from build123d import *
from build123d.topology import SkipClean

# Parameters (mm, degrees)
BOSS_EXTRUDE1_DEPTH                = 7.5
CUT_EXTRUDE1_REACH                 = 158.924
SKETCH2_W                          = 18
SKETCH2_H                          = 40
M5_CLEARANCE_HOLE1_D               = 5.8
CUT_EXTRUDE2_REACH                 = 158.924
F_7_0_7_DIAMETER_HOLE1_D           = 7
F_7_0_7_DIAMETER_HOLE1_DEPTH       = 20
MOVE_FACE1_BY                      = 0.6
SKETCH15_W                         = 15
SKETCH15_H                         = 15
BOSS_EXTRUDE3_DEPTH                = 10
M5_CLEARANCE_HOLE2_D               = 5.8
SKETCH19_W                         = 125
SKETCH19_H                         = 15
SKETCH19_R                         = 3.5
SKETCH19_R_2                       = 5
BOSS_EXTRUDE4_DEPTH                = 6
SKETCH23_R                         = 5
SKETCH23_R_2                       = 2.9
BOSS_EXTRUDE5_DEPTH                = 1
F_4_5_START                        = -7.5
F_4_5_4_5_DIAMETER_HOLE1_OUTLINE_R = 2.25
F_4_5_4_5_DIAMETER_HOLE1_DEPTH     = 15


# Read off the part's stored shape, not the designer's step: Ø4.5 (4.5) Diameter Hole1
with BuildPart() as part:
    # Sketch1 → Boss-Extrude1 (new, symmetric)
    with BuildSketch(Plane.XY):
        Polygon((0, 0), (120, 0), (0, -100), align=None)
    extrude(amount=BOSS_EXTRUDE1_DEPTH, both=True)

    # Sketch2 → Cut-Extrude1 (cut, up to next)
    with BuildSketch(Plane.XY.offset(7.5), mode=Mode.PRIVATE) as cut_extrude1_sk1:
        with Locations((9, -40)):
            Rectangle(SKETCH2_W, SKETCH2_H)
    cut_extrude1_tool1 = extrude(cut_extrude1_sk1.sketch, amount=-CUT_EXTRUDE1_REACH, mode=Mode.PRIVATE) & part.part
    add(cut_extrude1_tool1.solids().sort_by_distance((9, -40, 7.5))[0], mode=Mode.SUBTRACT)

    # M5 Clearance Hole1 (through all)
    with Locations(Plane(origin=(0, 0, 0), x_dir=(1, 0, 0), z_dir=(0, 1, 0))):
        with Locations((4.5, 0)):
            Hole(M5_CLEARANCE_HOLE1_D / 2)

    # Sketch8 → Cut-Extrude2 (cut, up to next)
    with BuildSketch(Plane.XY.offset(7.5), mode=Mode.PRIVATE) as cut_extrude2_sk1:
        Polygon((0, -70), (36, -70), (0, -100), align=None)
    cut_extrude2_tool1 = extrude(cut_extrude2_sk1.sketch, amount=-CUT_EXTRUDE2_REACH, mode=Mode.PRIVATE) & part.part
    add(cut_extrude2_tool1.solids().sort_by_distance((12, -80, 7.5))[0], mode=Mode.SUBTRACT)

    # Ø7.0 (7) Diameter Hole1
    with Locations(Plane(origin=(0, 0, 0), x_dir=(1, 0, 0), z_dir=(0, 1, 0))):
        with Locations((115, 0)):
            Hole(F_7_0_7_DIAMETER_HOLE1_D / 2, depth=F_7_0_7_DIAMETER_HOLE1_DEPTH)

    # Move Face1: a curved face moved inward by 0.6
    add(Solid.thicken(part.faces().sort_by_distance((7.4, -65, 0))[0], -MOVE_FACE1_BY), mode=Mode.SUBTRACT)

    # Sketch15 → Boss-Extrude3 (add)
    with BuildSketch(Plane.ZY):
        with Locations((0, -77.5)):
            Rectangle(SKETCH15_W, SKETCH15_H)
    extrude(amount=-BOSS_EXTRUDE3_DEPTH)

    # M5 Clearance Hole2 (through all)
    with Locations(Plane(origin=(10, 0, 0), x_dir=(0, 0, -1), z_dir=(1, 0, 0))):
        with Locations((0, -77.5)):
            Hole(M5_CLEARANCE_HOLE2_D / 2)

    # Sketch19 → Boss-Extrude4 (add)
    with SkipClean():  # the faces are left unmerged after this step: merging them gives an invalid solid
        with BuildSketch(Plane(origin=(0, 0, 0), x_dir=(1, 0, 0), z_dir=(0, 1, 0))):
            with Locations((57.5, 0)):
                Rectangle(SKETCH19_W, SKETCH19_H)
            with Locations(Location((115, 0, 0), (0, 0, 270))):
                Circle(SKETCH19_R, mode=Mode.SUBTRACT)
            with Locations(Location((4.5, 0, 0), (0, 0, 154.158067237))):
                Circle(SKETCH19_R_2, mode=Mode.SUBTRACT)
        extrude(amount=BOSS_EXTRUDE4_DEPTH)

    # Sketch23 → Boss-Extrude5 (add)
    with BuildSketch(Plane(origin=(0, 0, 0), x_dir=(1, 0, 0), z_dir=(0, 1, 0))):
        with Locations(Location((4.5, 0, 0), (0, 0, 270))):
            Circle(SKETCH23_R)
        with Locations(Location((4.5, 0, 0), (0, 0, 270))):
            Circle(SKETCH23_R_2, mode=Mode.SUBTRACT)
    extrude(amount=BOSS_EXTRUDE5_DEPTH)

    # Ø4.5 (4.5) Diameter Hole1 outline → Ø4.5 (4.5) Diameter Hole1 (cut)
    with BuildSketch(Plane.XY.offset(F_4_5_START)):
        with Locations((91, -4)):
            Circle(F_4_5_4_5_DIAMETER_HOLE1_OUTLINE_R)
        with Locations((28, -57)):
            Circle(F_4_5_4_5_DIAMETER_HOLE1_OUTLINE_R)
        with Locations((28, -4)):
            Circle(F_4_5_4_5_DIAMETER_HOLE1_OUTLINE_R)
    extrude(amount=F_4_5_4_5_DIAMETER_HOLE1_DEPTH, mode=Mode.SUBTRACT)


solid = part.part
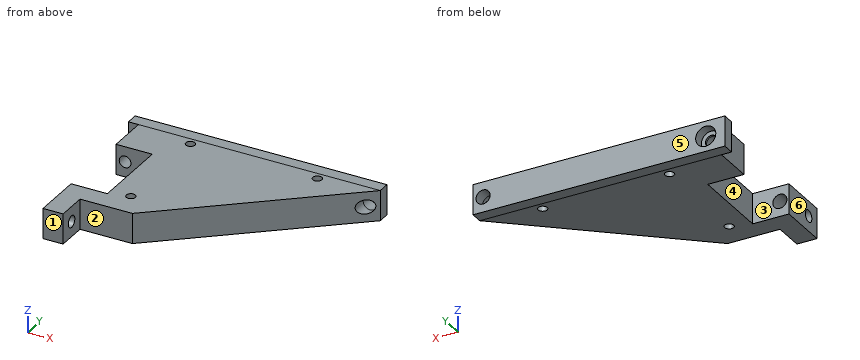
Can you work these out from the model? Positions are in its coordinate system, mm. Face numbers are marked on the shaded views. A direction names the side the tool comes from. Coordinates: 2 decimals unless noted, no trailing zeros. Loops run counter-clockwise (first coordinate to the right, second up) from the corner with the lowest first, then second, coordinate; pieces in that order, holes last. Notation, with made-up numbers: (53.25, -39.75) - (65.25, -39.75) arc R17 cw to (65.25, -17.75) - close; hole circle Ø5 at (-39, -29). An arc over 180 degrees is marked (long way). Put each result on its own line as item: value. Start each with the question number.
Item 1: Suppose I cut it at C-C (x = 3). Please give me the cut outline in (y, z), and give its area (3 significant figures).
Item 2: Suppose I cut it at B-B (x = 28). Please give me the cut outline in (y, z).
Item 3: If I drill on line 1 along X through (y, z) = (0.8, 0); line 2 along Y through (x, z) = (7, -5.25); line 3 along Z through (x, y) = (4.5, 4.75), over which ranges is the centre line in solid material (lowest first)?
Item 4: If we mould it in two halves opening along Y, with no side actions, what happens to the marked faces 3, 4, 5 and 6? For each: +Y half, -Y half, draft (parallel to the pull), parting line (faces both ways), or undercut.
Item 5: Which directions (+Z, -Z, +X, -X, +Y, -Y) give clear straight access to the entire face, cutting with the end or side of a thin tool? Please do the marked faces 1 and 2.
Item 6: Suppose I cut it at A-A (y = -57). Please give me the cut outline in (x, z), and give its area (4 significant figures).
Item 7: For pin 1 (4.5 mm diameter, centred on y = -76, z = 1, fed in from -X); pin 2 (3 mm diameter, centred on y = -75.5, z = 1.5, fed in from +X); pin 3 (1 mm diameter, centred on y = -70, z = 2.5, fed in from +X), each with a flat end and sliding along its axis, tell me the tip position at first contact or that it passes through.
Item 8: Suppose I cut it at D-D (z = 0). State how many separate pieces and enclosed holes the cut face has, and give its area (3 significant figures).
Here are the results:
1. outline: (-85, -7.5) - (-60, -7.5) - (-60, -3.16) - (-70, -3.16) - (-70, 3.16) - (-60, 3.16) - (-60, 7.5) - (-85, 7.5) - close; (-20, -7.5) - (6, -7.5) - (6, -4.77) - (1, -4.77) - (1, -2.48) - (-20, -2.48) - close; (-20, 2.48) - (1, 2.48) - (1, 4.77) - (6, 4.77) - (6, 7.5) - (-20, 7.5) - close; hole circle Ø5.8 at (-77.5, 0)
1. area: 523 mm²
2. outline: (-70, -7.5) - (-59.25, -7.5) - (-59.25, 7.5) - (-70, 7.5) - close; (-54.75, -7.5) - (-6.25, -7.5) - (-6.25, 7.5) - (-54.75, 7.5) - close; (-1.75, -7.5) - (6, -7.5) - (6, 7.5) - (-1.75, 7.5) - close
3. line 1: -5 to 1.6, 7.4 to 111.5, 118.5 to 120
3. line 2: -85 to -60, -20 to 6
3. line 3: -7.5 to -5, 5 to 7.5
4. face 3: undercut
4. face 4: undercut
4. face 5: +Y half
4. face 6: draft
5. face 1: +Z, -Z, +X, -X, -Y
5. face 2: +Z, -Z, +X, -Y
6. outline: (18, -7.5) - (25.75, -7.5) - (25.75, 7.5) - (18, 7.5) - close; (30.25, -7.5) - (51.6, -7.5) - (51.6, 7.5) - (30.25, 7.5) - close
6. area: 436.5 mm²
7. pin 1: x = 0
7. pin 2: x = 10
7. pin 3: x = 36.6
8. separate pieces: 4
8. enclosed holes: 3
8. area: 5,220 mm²
